Autodesk Inventor part; units mm, degrees
ref_plane "YZ Plane" through (0, 0, 0) normal (1, 0, 0) x (0, 1, 0)
ref_plane "XZ Plane" through (0, 0, 0) normal (0, 1, 0) x (-1, 0, 0)
ref_plane "XY Plane" through (0, 0, 0) normal (0, 0, 1) x (1, 0, 0)
sketch "Sketch1" plane through (0, 0, 0) normal (0, 0, 1) x (1, 0, 0)
  circle A0 centre (0, 0) radius 10
  circle A1 centre (0, 0) radius 15
  line L0 (0, 15) -> (50, 15)
  line L1 (50, 15) -> (50, -15)
  line L2 (0, -15) -> (50, -15)
  line L3 (-15, 0) -> (50, 0)
  point P0 (-10, 0)
  point P1 (10, 0)
  dimension "d0" = 20
  dimension "d1" = 30
  dimension "d2" = 50
extrude "Extrusion1" add sketch "Sketch1" along normal blind 30 contours A0 L3 A1 | A1 L0 L1 L3 picked at (13.208, 1.1126)
sketch "Sketch2" plane through (50, 0, 0) normal (1, 0, 0) x (0, 0, -1)
  line L0 (0, 0) -> (-30, 0)
  circle A0 centre (-15, 0) radius 10
  point P0 (-25, 0)
  point P1 (-5, 0)
  dimension "d5" = 20
extrude "Extrusion2" cut sketch "Sketch2" against normal blind 20 contours L0 A0 picked at (-12.505, 2.2104)
sketch "Sketch3" plane through (0, 15, 0) normal (0, 1, 0) x (1, 0, 0)
  line L0 (50, 0) -> (0, 0)
  line L1 (0, 0) -> (0, -30)
  line L2 (50, -30) -> (0, -30)
  line L3 (50, 0) -> (50, -30)
  line L4 (50, -5) -> (50, -25) construction
  line L5 (50, -15) -> (40, -15) construction
  circle A0 centre (40, -15) radius 5
  dimension "d8" = 10
  dimension "d9" = 10
ref_plane "Work Plane1" through (0, 0, 15) normal (0, 0, 1) x (1, 0, 0)
extrude "Extrusion3" cut sketch "Sketch3" against normal blind 10 contours A0
properties part number "AbrazaderaBarraAscenso1"
CAD build for the part. Positions are in the model's coordinates, mm. A direction names the side the tool comes from. Coordinates: 2 decimals unless noted, no trailing zeros. Order: outer loops, then holes, each group sorted by start corner. A loop starts at its lowest first (then second) coordinate and runs counter-clockwise, first axis right, second up. Notation, with made-up numbers: (-10.75, 4) - (3.25, 4) arc R27 ccw to (3.25, 22) - close; hole circle Ø4 at (-34, 69). An arc over 180 degrees is marked (long way). Answer in a Markdown table with one row per item.
1. Drill centre lines: L1, parallel to Z at x = 40, y = 13.75; L2, parallel to Z at x = 38, y = 0.5; L3, parallel to X at y = 11, z = 15. Where is each one in solid material? Low to high. Write a range as from..to.
Answer:
| item | result |
|---|---|
| L1 | 0..10, 20..30 |
| L2 | 0..5.01, 24.99..30 |
| L3 | -10.2..35, 45..50 |
2. Slice it at A-A, the plane z = 15. List the corners of the cut face in (x, y).
Answer:
| item | result |
|---|---|
| outline | (-15, 0) - (-10, 0) arc R10 cw to (10, 0) - (30, 0) - (30, 10) - (35, 10) - (35, 15) - (0, 15) arc R15 ccw to start; (45, 10) - (50, 10) - (50, 15) - (45, 15) - close |
3. Pull direction Z, two halves, no side cores. Call faces 1 (the face through (24, 8, 30)), 2 (the face through (-13, 0, 15)), 3 (the face through (30, 4, 15)): +Z half, -Z half, draft (parallel to the pull), parting line (faces both ways), or undercut.
Answer:
| item | result |
|---|---|
| face 1 | +Z half |
| face 2 | draft |
| face 3 | undercut |
4. Slice it at D-D, the plane y = 12. List the corners of the cut face in (x, z), then the cut area to 3 significant figures.
Answer:
| item | result |
|---|---|
| outline | (-9, 0) - (50, 0) - (50, 30) - (-9, 30) - close; hole circle Ø10 at (40, 15) |
| area | 1,690 mm² |
5. Flat gauge pins, fed straight in: P1, Ø4, axis at x = 20.5, z = 5.5, coming from the -Y side; P2, Ø3, axis at y = 10.5, z = 15, coming from the -X side; P3, Ø1.5, axis at x = 37.5, z = 10.5, coming from the -Y side; P4, Ø6, axis at x = 40, z = 15, coming from the -Y side. Where does each tip first touch, or does it go through?
Answer:
| item | result |
|---|---|
| P1 | y = 0 |
| P2 | x = -12 |
| P3 | y = 8.51 |
| P4 | through |
6. Slice it at B-B, the plane y = 6.75. List the corners of the cut face in (x, z).
Answer:
| item | result |
|---|---|
| outline | (-13.4, 0) - (-7.38, 0) - (-7.38, 30) - (-13.4, 30) - close; (7.38, 0) - (50, 0) - (50, 7.62) - (30, 7.62) - (30, 22.38) - (50, 22.38) - (50, 30) - (7.38, 30) - close |
7. 3-axis set-ups, long thin cutter, end or side, ignore diameter. For faces 4 (the face through (35.7, 9.32, 11.37)), 5 (the face through (25, 0, 15)): which of +Z, -Z, +X, -X, +Y, -Y reach the whole face in a straight line?
Answer:
| item | result |
|---|---|
| face 4 | +X, -Y |
| face 5 | +Z, -Z, +X, -X, -Y |
8. Slice it at C-C, the plane x = 33.5. List the corners of the cut face in (y, z).
Answer:
| item | result |
|---|---|
| outline | (0, 0) - (15, 0) - (15, 30) - (0, 30) - (0, 25) arc R10 cw to (0, 5) - close |
